Autodesk Inventor part; units mm, degrees
ref_plane "YZ Plane" through (0, 0, 0) normal (1, 0, 0) x (0, 1, 0)
ref_plane "XZ Plane" through (0, 0, 0) normal (0, 1, 0) x (-1, 0, 0)
ref_plane "XY Plane" through (0, 0, 0) normal (0, 0, 1) x (1, 0, 0)
sketch "Sketch1" plane through (0, 0, 0) normal (0, 1, 0) x (-1, 0, 0)
  arc A0 (-17.5636, 5.8132) -> (-8.5833, 9.5329) centre (-17.5636, 18.5132) ccw
  arc A1 (-17.5636, 5.8132) -> (-8.5833, 9.5329) centre (-17.5636, 18.5132) ccw
  arc A2 (-8.5833, -9.3366) -> (-17.5636, -5.6168) centre (-17.5636, -18.3168) ccw
  arc A3 (-8.5833, -9.3366) -> (-17.5636, -5.6168) centre (-17.5636, -18.3168) ccw
  line L0 (-17.5636, 5.8132) -> (-17.5636, -5.6168)
  line L1 (-8.5833, 9.5329) -> (11.8765, 9.5329)
  line L2 (-8.5833, -9.3366) -> (11.1934, -9.3366)
  arc A4 (11.8765, 6.0101) -> (11.8765, -5.8137) centre (18.8929, 0.0982) ccw
  line L3 (11.8765, -9.3366) -> (11.1934, -9.3366)
  line L4 (11.8765, 9.5329) -> (11.8765, 6.0101)
  line L5 (11.8765, -5.8137) -> (11.8765, -9.3366)
  circle A5 centre (5.9079, 5.8536) radius 1.8
  circle A6 centre (5.9079, 5.8536) radius 1.8
  circle A7 centre (-4.2521, 5.8536) radius 1.8
  circle A8 centre (-4.2521, 5.8536) radius 1.8
  circle A9 centre (5.9079, -5.6573) radius 1.8
  circle A10 centre (5.9079, -5.6573) radius 1.8
  circle A11 centre (-4.2521, -5.6573) radius 1.8
  circle A12 centre (-4.2521, -5.6573) radius 1.8
  point P0 (12.4052, 6.5859)
extrude "Extrusion1" add sketch "Sketch1" along normal blind 4.445
sketch "Sketch2" plane through (0, 4.445, 0) normal (0, 1, 0) x (1, 0, 0)
  line L0 (-11.8765, -9.5329) -> (8.5833, -9.5329)
  line L1 (8.5833, 9.3366) -> (-11.8765, 9.3366)
  line L2 (0, -9.5329) -> (-2.54, -9.5329)
  line L3 (-2.54, 9.3366) -> (0, 9.3366)
  line L4 (0, 9.3366) -> (0, -9.5329)
  line L5 (-2.54, -1.3682) -> (-9.8062, -1.3682)
  line L6 (-2.54, 1.1718) -> (-9.8062, 1.1718)
  arc A0 (-11.8765, -6.0101) -> (-11.8765, 5.8137) centre (-18.8929, -0.0982) ccw
  arc A1 (-9.8062, -1.3682) -> (-9.8062, 1.1718) centre (-18.8929, -0.0982) ccw
  line L7 (-2.54, -9.5329) -> (-2.54, -1.3682)
  line L8 (-2.54, 1.1718) -> (-2.54, 9.3366)
  point P0 (0, 0)
  dimension "d2" = 2.54
extrude "Extrusion2" add sketch "Sketch2" along normal blind 11.43
sketch "Sketch3" plane through (0, 4.445, 0) normal (0, 1, 0) x (1, 0, 0)
  line L0 (0, -11.1934) -> (18.2988, -11.1934)
  line L1 (18.2988, -11.1934) -> (18.2988, 11.7125)
  line L2 (18.2988, 11.7125) -> (0, 11.7125)
  line L3 (0, 11.7125) -> (0, -11.1934)
  point P0 (0, 0)
extrude "Extrusion3" cut sketch "Sketch3" against normal blind 1.27
sketch "Sketch4" plane through (0, 15.875, 0) normal (0, 1, 0) x (1, 0, 0)
  arc A0 (20.271, 9.3366) -> (20.3081, -9.5329) centre (70.2056, 0) ccw
  line L0 (8.5833, -9.5329) -> (0, -9.5329)
  line L1 (-11.8765, -6.0101) -> (-11.8765, -9.5329)
  line L2 (7.4252, -9.5329) -> (-11.8765, -9.5329)
  line L3 (-11.8765, -9.5329) -> (-11.8765, -6.0101)
  arc A1 (-11.8765, -6.0101) -> (-11.8765, 5.8137) centre (-18.8929, -0.0982) ccw
  line L4 (-11.8765, 9.3366) -> (-11.8765, 5.8137)
  line L5 (-11.8765, 5.8137) -> (-11.8765, 9.3366)
  line L6 (-11.8765, 9.3366) -> (7.3957, 9.3366)
  line L7 (0, 9.3366) -> (8.5833, 9.3366)
  arc A2 (-11.8765, -6.0101) -> (-11.8765, 5.8137) centre (-18.8929, -0.0982) ccw
  line L8 (-11.8765, -9.5329) -> (8.5833, -9.5329)
  line L9 (-11.8765, -9.5329) -> (20.3081, -9.5329)
  line L10 (8.5833, 9.3366) -> (-11.8765, 9.3366)
  line L11 (-11.8765, 9.3366) -> (20.271, 9.3366)
  circle A3 centre (-5.9079, -5.8536) radius 1.8
  circle A4 centre (-5.9079, -5.8536) radius 1.8
  circle A5 centre (-5.9079, 5.6573) radius 1.8
  circle A6 centre (-5.9079, 5.6573) radius 1.8
  circle A7 centre (4.2521, -5.8536) radius 1.8
  circle A8 centre (4.2521, -5.8536) radius 1.8
  circle A9 centre (4.2521, 5.6573) radius 1.8
  circle A10 centre (4.2521, 5.6573) radius 1.8
  circle A11 centre (14.4121, -0.0982) radius 1.8
  point P0 (0, 0)
  dimension "d10" = 101.6
  dimension "d13" = 3.6
extrude "Extrusion4" add sketch "Sketch4" along normal blind 4.445
sketch "Sketch5" plane through (0, 20.32, 0) normal (0, 1, 0) x (1, 0, 0)
  line L0 (0, -9.5329) -> (20.3081, -9.5329)
  line L1 (20.3081, -9.5329) -> (0, -9.5329)
  line L2 (0, -9.5329) -> (0, 9.3366)
  line L3 (0, -9.5329) -> (0, 9.3366)
  line L4 (20.271, 9.3366) -> (0, 9.3366)
  line L5 (0, 9.3366) -> (20.271, 9.3366)
  arc A0 (20.271, 9.3366) -> (20.3081, -9.5329) centre (70.2056, 0) ccw
  circle A1 centre (4.2521, -5.8536) radius 1.8
  circle A2 centre (4.2521, -5.8536) radius 1.8
  circle A3 centre (4.2521, 5.6573) radius 1.8
  circle A4 centre (4.2521, 5.6573) radius 1.8
  circle A5 centre (14.4121, -0.0982) radius 1.8
  circle A6 centre (14.4121, -0.0982) radius 1.8
  point P0 (0, 0)
extrude "Extrusion5" cut sketch "Sketch5" against normal blind 2.2225
fillet "Fillet1" radius 3.175 2 edges at (-2.54, 10.16, 1.3682) (-2.54, 10.16, -1.1718)
sketch "Sketch6" plane through (0, 20.32, 0) normal (0, 1, 0) x (1, 0, 0)
  circle A0 centre (-5.9079, -5.8536) radius 1.8
  circle A1 centre (-5.9079, -5.8536) radius 1.8
  circle A2 centre (-5.9079, 5.6573) radius 1.8
  circle A3 centre (-5.9079, 5.6573) radius 1.8
  circle A4 centre (4.2521, -5.8536) radius 1.8
  circle A5 centre (4.2521, -5.8536) radius 1.8
  circle A6 centre (4.2521, 5.6573) radius 1.8
  circle A7 centre (4.2521, 5.6573) radius 1.8
  circle A8 centre (14.4121, -0.0982) radius 1.8
  circle A9 centre (14.4121, -0.0982) radius 1.8
  line L0 (-11.8765, -9.5329) -> (-2.54, -9.5329)
  arc A10 (20.271, 9.3366) -> (20.3081, -9.5329) centre (70.2056, 0) ccw
  line L1 (-11.8765, -9.5329) -> (20.3081, -9.5329)
  line L2 (-11.8765, -6.0101) -> (-11.8765, -9.5329)
  line L3 (-11.8765, -9.5329) -> (-11.8765, -6.0101)
  line L4 (-11.8765, 9.3366) -> (-11.8765, 5.8137)
  line L5 (-11.8765, 5.8137) -> (-11.8765, 9.3366)
  line L6 (0, 9.3366) -> (20.271, 9.3366)
  line L7 (-11.8765, 9.3366) -> (20.271, 9.3366)
  arc A11 (-11.8765, -6.0101) -> (-11.8765, 5.8137) centre (-18.8929, -0.0982) ccw
  line L8 (0, -9.5329) -> (0, 9.3366)
  line L9 (8.5833, 9.3366) -> (-11.8765, 9.3366)
  point P0 (0, 0)
properties part number "MountingBracket"
Can you work these out from the model? Positions are in its coordinate system, mm. A direction names the side the tool comes from. Round coordinates to 2 decimals unless told otherwise and drop trailing zeros. Loops run counter-clockwise (first coordinate to the right, second up) from the corner with the lowest first, then second, coordinate; pieces in that order, holes last. Notation, with made-up numbers: (-32, 16) - (20, 16) arc R20 cw to (20, 42) - close; hole circle Ø8 at (-32, 15.25). An arc over 180 degrees is marked (long way). Use CSV: the item, a comma, the result in double quotes. Start each with the question number.
1) For pin 1 Ø8 at (x, z) = (8, -6) entering from +Y; pin 2 Ø2 at (x, y) = (-9, 12) entering from -Z; pin 3 Ø2.5 at (y, z) = (8.5, 6.5) entering from -X, each with a flat end and sliding along its axis, tell me the tip position at first contact or that it passes through.
2) If we section it at C-C on z = 1: Write out the boundary of the cut face in (x, y) (1 decimal).
3) If we section it at B-B on z = -6.5: Count the separate pieces of the cut face and the enclosed holes in it, plus the area to 3 significant figures.
4) Please list where these lines run through material, in increasing order: probe 1 along Y at (x, z) = (-7.5, 8) (3 decimals); probe 2 along Y at (x, z) = (2, -2.5) (1 decimal); probe 3 along Z at (x, y) = (-7, 1.25). Write a range as [from, to].
5) For faces 4 (the flat face through (-8, 15.875, -5)), 5 (the flat face through (0, 19, 0)), 6 (the flat face through (-2.54, 10, 7)), 7 (the flat face through (9, 3.175, 0)), 8 (the cylindrical face through (12.639, 1.565, 6.807)), which set-ups out of +Z, -Z, +X, -X, +Y, -Y let a thin tool reach every point of the face, with its end or its side?
6) If we section it at A-A on x = 8: Write out the boundary of the cut face in (y, z) (1 decimal).
7) If we section it at D-D on y = 16.5: Write out the boundary of the cut face in (x, z), plus the area to 3 significant figures.
8) We'd pull the mould along X, two halves only. Please class faces 1 (the cylindrical face through (-3.45, 10.24, 2.32)), 2 (the cylindrical face through (-6.876, 2.191, -7.175)), 3 (the flat face through (-8, 4.445, 6)): released by +X, released by -X, zero draft, split by the parting line, or undercut.
Geometry results:
1,pin 1,"stops at y = 18.1"
1,pin 2,"stops at z = -1.17"
1,pin 3,"stops at x = -2.54"
2,outline,"(-9.8, 0) - (17.6, 0) - (17.6, 3.2) - (0, 3.2) - (0, 15.9) - (12.9, 15.9) - (12.9, 18.1) - (0, 18.1) - (0, 20.3) - (-9.8, 20.3) - close; (16, 15.9) - (19.4, 15.9) - (19.4, 18.1) - (16, 18.1) - close"
3,separate pieces,"5"
3,enclosed holes,"0"
3,area,"174 mm2"
4,probe 1,"y = [0, 4.445], [15.875, 20.32]"
4,probe 2,"y = [0, 3.2], [15.9, 18.1]"
4,probe 3,"z = [-9.34, -7.09], [-4.23, 4.42], [7.28, 9.53]"
5,face 4,"-Z, -X"
5,face 5,"+Z, -Z, +X, +Y"
5,face 6,"+Z, -X"
5,face 7,"+Z, -Z, +X"
5,face 8,"+Z, +X, -Y"
6,outline,"(0, -9.3) - (3.2, -9.3) - (3.2, 9.5) - (0, 9.5) - close; (15.9, -9.3) - (18.1, -9.3) - (18.1, 9.5) - (15.9, 9.5) - close"
7,outline,"(-11.88, -9.34) - (20.27, -9.34) arc R50.8 cw to (20.31, 9.53) - (-11.88, 9.53) - (-11.88, 6.01) arc R9.17 cw to (-11.88, -5.81) - close; hole circle Ø3.6 at (-5.91, -5.66); hole circle Ø3.6 at (-5.91, 5.85); hole circle Ø3.6 at (4.25, -5.66); hole circle Ø3.6 at (4.25, 5.85); hole circle Ø3.6 at (14.41, 0.1)"
7,area,"527 mm2"
8,face 1,"released by -X"
8,face 2,"undercut"
8,face 3,"zero draft"
